```python
from build123d import *

# Parameters (mm, degrees)
SKETCH_R         = 10.2
PAD_DEPTH        = 8
SKETCH002_W      = 8
SKETCH002_H      = 3.8
PAD001_DEPTH     = 8
SKETCH003_W      = 8
SKETCH003_H      = 9
PAD002_DEPTH     = 8
POCKET_DEPTH     = 8.001
SKETCH005_R      = 1.6
POCKET001_DEPTH  = 12.101
HOLE_D           = 3.2
HOLE_CSINK_D     = 6
HOLE_CSINK_ANGLE = 90
POCKET003_DEPTH  = 2
FILLET_R         = 3.9
FILLET001_R      = 1


with BuildPart() as part:
    # Sketch → Pad (new body)
    with BuildSketch(Plane.XY):
        Circle(SKETCH_R)
    extrude(amount=PAD_DEPTH)

    # Sketch002 → Pad001 (join)
    with BuildSketch(Plane.XY):
        with Locations((-14.021477, 0)):
            Rectangle(SKETCH002_W, SKETCH002_H)
    extrude(amount=PAD001_DEPTH)

    # Sketch003 → Pad002 (join)
    with BuildSketch(Plane.XY):
        with Locations((13.153688, 0)):
            Rectangle(SKETCH003_W, SKETCH003_H)
    extrude(amount=PAD002_DEPTH)

    # Sketch004 (on Face10 of Pad002) → Pocket (cut, through all)
    with BuildSketch(Plane.XY.offset(8)):
        with BuildLine():
            ThreePointArc((6.179806, 0.5), (-6.2, 0), (6.179806, -0.5))
            Line((6.179806, -0.5), (17.153688, -0.5))
            Line((17.153688, -0.5), (17.153688, 0.5))
            Line((6.179806, 0.5), (17.153688, 0.5))
        make_face()
    extrude(amount=-POCKET_DEPTH, mode=Mode.SUBTRACT)

    # Sketch005 (on Face7 of Pocket) → Pocket001 (cut, through all)
    with BuildSketch(Plane.XZ.offset(1.9)):
        with Locations((-14.021477, 4)):
            Circle(SKETCH005_R)
    extrude(amount=-POCKET001_DEPTH, mode=Mode.SUBTRACT)

    # Hole (through all)
    with Locations(Plane.XZ.offset(4.5)):
        with Locations((13.153688, 4)):
            CounterSinkHole(HOLE_D / 2, HOLE_CSINK_D / 2, counter_sink_angle=HOLE_CSINK_ANGLE)

    # Sketch007 → Pocket003 (cut)
    with BuildSketch(Plane(origin=(0, 4.5, 0), x_dir=(-1, 0, 0), z_dir=(0, 1, 0))):
        Polygon((-9.805056, 4), (-11.479372, 6.9), (-14.828004, 6.9), (-16.502319, 4), (-14.828004, 1.1), (-11.479372, 1.1), align=None)
    extrude(amount=-POCKET003_DEPTH, mode=Mode.SUBTRACT)

    # Fillet
    fillet_edges = [part.edges().sort_by_distance(p)[0] for p in [
        (-18.021477, 0, 8),
        (-18.021477, 0, 0),
    ]]
    fillet(fillet_edges, radius=FILLET_R)

    # Fillet001
    fillet001_edges = [part.edges().sort_by_distance(p)[0] for p in [
        (9.153688, 4.5, 4),
        (9.153688, -4.5, 4),
        (-10.021477, -1.9, 4),
        (-10.021477, 1.9, 4),
        (6.179806, -0.5, 4),
        (6.179806, 0.5, 4),
    ]]
    fillet(fillet001_edges, radius=FILLET001_R)


solid = part.part
```
Design review of the part built by this model. Coordinates are the model's own, in mm. A direction names the side the tool comes from. Round coordinates to 2 decimals unless told otherwise and drop trailing zeros. Write each loop counter-clockwise with the first axis right and the second up, starting at its lowest first coordinate (ties: lowest second). Pieces come first, ordered by that corner, then holes. Notation, with made-up numbers: (29, -1) -> (50, -1) arc R13 ccw to (50, 9) -> close; hole circle Ø1 at (62.25, 8.5). An arc over 180 degrees is marked (long way). Answer in a Markdown table with one row per item.
Q1. Take a section at C-C, the plane x = -15. State the section outline as (y, z) points, then the cut area to 3 significant figures.
The answers:
| item | result |
|---|---|
| outline | (-1.9, 0.1) -> (1.9, 0.1) -> (1.9, 2.73) -> (-1.9, 2.73) -> close; (-1.9, 5.27) -> (1.9, 5.27) -> (1.9, 7.9) -> (-1.9, 7.9) -> close |
| area | 20.0 mm² |
Q2. Clearance check with flat-ended pins moving along their axes: pin 1 Ø3.5 at (x, z) = (13.5, 2) entering from +Y; pin 2 Ø4 at (x, z) = (13.15, 4) entering from -Y; pin 3 Ø4 at (x, z) = (-14.02, 4) entering from -Y. State where each tip first meets the part, or that it passes through.
The answers:
| item | result |
|---|---|
| pin 1 | y = 4.5 |
| pin 2 | y = -3.5 |
| pin 3 | y = -1.9 |
Q3. Take a section at B-B, the plane x = 0. State the section outline as (y, z) points.
The answers:
| item | result |
|---|---|
| outline | (-10.2, 0) -> (-6.2, 0) -> (-6.2, 8) -> (-10.2, 8) -> close; (6.2, 0) -> (10.2, 0) -> (10.2, 8) -> (6.2, 8) -> close |
Q4. Take a section at D-D, the plane y = -7. State the section outline as (x, z) points.
The answers:
| item | result |
|---|---|
| outline | (-7.42, 0) -> (7.42, 0) -> (7.42, 8) -> (-7.42, 8) -> close |
Q5. Draft analysis for pull direction X (two halves, no side actions). For faces 5 (the face through (10.63, 3.51, 5.43)), 6 (the face through (17.154, 2, 4)), 7 (the face through (11, -0.5, 4)), 8 (the face through (-10.22, 2.1, 4.06)), state which applies: +X half, -X half, draft (parallel to the pull), parting line (faces both ways), or undercut.
The answers:
| item | result |
|---|---|
| face 5 | undercut |
| face 6 | +X half |
| face 7 | draft |
| face 8 | -X half |
Q6. For faces 1 (the face through (6.405, -0.729, 3.944)), 2 (the face through (-14, 1.9, 6)), 3 (the face through (16, 4.5, 2)), 4 (the face through (13, 4, 1.1)), list the 3-axis set-ups (+Z, -Z, +X, -X, +Y, -Y) from which the entire face can be reached by the end or side of a thin tool; tool diameter is ignored.
The answers:
| item | result |
|---|---|
| face 1 | +Z, -Z |
| face 2 | +Z, -Z, -X, +Y |
| face 3 | +Z, -Z, +X, +Y |
| face 4 | +Y |
Q7. Take a section at A-A, the plane y = 0. State the section outline as (x, z) points, then the cut area to 3 significant figures.
The answers:
| item | result |
|---|---|
| outline | (-18.02, 3.9) arc R3.9 ccw to (-14.12, 0) -> (-6.2, 0) -> (-6.2, 8) -> (-14.12, 8) arc R3.9 ccw to (-18.02, 4.1) -> close; hole circle Ø3.2 at (-14.02, 4) |
| area | 80.0 mm² |
Q8. To check wall thickness, follow L1, parallel to X at y = 3.5, z = 1.75; L2, parallel to X at y = 4, z = 4.75; L3, parallel to Y at x = 0, z = 4.75. State the ranges of each line that lie inside material, in increasing order. Write a range as [from, to].
The answers:
| item | result |
|---|---|
| L1 | [-9.58, -5.12], [5.12, 11.1], [15.2, 17.15] |
| L2 | [-9.38, -4.74], [4.74, 10.24], [16.07, 17.15] |
| L3 | [-10.2, -6.2], [6.2, 10.2] |
